Geometry: final body of the model. Coordinates: model frame, mm. A direction names the side the tool comes from. Round coordinates to 2 decimals unless told otherwise and drop trailing zeros. Write each loop counter-clockwise with the first axis right and the second up, starting at its lowest first coordinate (ties: lowest second). Pieces come first, ordered by that corner, then holes. Notation, with made-up numbers: M -28.5,22.25 L 8.5,22.25 A27 cw 8.5,61.25 Z; hole C 31.5,30.5 d2. An arc over 180 degrees is marked long. Answer as CSV lines item,"result". Start each with the question number.
Q1. Section query C-C on x = 1090.5. Output: boundary loops of the cut face in (y, z).
Q2. Reachability of faces 4 (the flat face through (1375, 624, -386)), 5 (the flat face through (419, -337, 0)), 6 (the flat face through (228, -460, -177)) from +Z, -Z, +X, -X, +Y, -Y: full face, straight path, thin tool, end or side. Return the list, or none.
Q3. Ray query, probe 1 along Y at (x, z) = (951.5, 916); probe 2 along X at (y, z) = (24, -425); probe 3 along Y at (x, z) = (288.5, -233). Return the intervals inside material, ascending.
Q4. First-contact query: pin 1 (1 mm diameter, centred on x = 1203, z = 115.5, fed in from +Y); pin 2 (12 mm diameter, centred on x = 274, y = -205.5, fed in from +Z); pin 3 (12 mm diameter, centred on x = 1136.5, y = 178.5, fed in from +Z). Flat tips, straight axial feed; report the tip coordinate or a pass-through.
Q5. Mould query, pull axis Y, two halves, no side actions, for faces 1 (the flat face through (248, -350, -350)), 2 (the flat face through (865, 40, -76)), 3 (the flat face through (1324, -710, -424)). Classes: pulls with the +Y half, pulls with the -Y half, needs draft (parallel to the pull), parting line crosses it, or undercut.
Q6. Section query B-B on x = 1325. Give the number of separate pieces and of enclosed holes in the cut face, and give its area (3 significant figures).
Q7. Section query A-A on z = 275. Output: boundary loops of the cut face in (x, y), and give its area (3 significant figures).
Q8. Section query D-D on z = -222. Output: boundary loops of the cut face in (x, y), and give its area (3 significant figures).
```python
from build123d import *

# Parameters (mm, degrees)
BOSS_EXTRUDE1_DEPTH = 40
SKETCH3_W           = 450
SKETCH3_H           = 500
SKETCH3_W_2         = 500
SKETCH3_H_2         = 450
BOSS_EXTRUDE2_DEPTH = 710
SKETCH5_W           = 410
SKETCH5_H           = 710
CUT_EXTRUDE1_DEPTH  = 150
SKETCH7_R           = 30
CUT_EXTRUDE2_DEPTH  = 150
SKETCH8_W           = 370
SKETCH8_H           = 670
CUT_EXTRUDE3_DEPTH  = 310
SKETCH9_W           = 370
SKETCH9_H           = 670
CUT_EXTRUDE4_DEPTH  = 460
SKETCH10_W          = 150
SKETCH10_H          = 150
BOSS_EXTRUDE3_DEPTH = 710
SKETCH11_W          = 310
SKETCH11_H          = 20
BOSS_EXTRUDE4_DEPTH = 410
SKETCH12_W          = 370
SKETCH12_H          = 670
CUT_EXTRUDE5_DEPTH  = 40
BOSS_EXTRUDE5_DEPTH = 370
SKETCH14_W          = 370
SKETCH14_H          = 670
CUT_EXTRUDE10_DEPTH = 40
BOSS_EXTRUDE6_DEPTH = 650
SKETCH17_W          = 175
SKETCH17_H          = 20
BOSS_EXTRUDE7_DEPTH = 1350


with BuildPart() as part:
    # Sketch2 → Boss-Extrude1 (new body)
    with BuildSketch(Plane(origin=(0, 0, 0), x_dir=(1, 0, 0), z_dir=(0, 1, 0))):
        Polygon((0, 500), (1400, 500), (900, 0), (0, 0), align=None)
        Polygon((900, 0), (1400, 500), (1400, 0), (1400, -1000), (900, -1000), align=None)
    extrude(amount=BOSS_EXTRUDE1_DEPTH)

    # Sketch3 → Boss-Extrude2 (add)
    with BuildSketch(Plane.XZ):
        with Locations((225, -250)):
            Rectangle(SKETCH3_W, SKETCH3_H)
        with Locations((1150, 775)):
            Rectangle(SKETCH3_W_2, SKETCH3_H_2)
    extrude(amount=BOSS_EXTRUDE2_DEPTH)

    # Sketch5 → Cut-Extrude1 (cut)
    with BuildSketch(Plane(origin=(0, 0, -500), x_dir=(-1, 0, 0), z_dir=(0, 0, -1))):
        with Locations((-245, -355)):
            Rectangle(SKETCH5_W, SKETCH5_H)
    extrude(amount=-CUT_EXTRUDE1_DEPTH, mode=Mode.SUBTRACT)

    # Sketch7 → Cut-Extrude2 (cut)
    with BuildSketch(Plane.XZ):
        with Locations(Location((115, -425, 0), (0, 0, 270))):
            Circle(SKETCH7_R)
        with Locations(Location((675, -425, 0), (0, 0, 270))):
            Circle(SKETCH7_R)
        with Locations(Location((1325, 275, 0), (0, 0, 270))):
            Circle(SKETCH7_R)
    extrude(amount=-CUT_EXTRUDE2_DEPTH, mode=Mode.SUBTRACT)

    # Sketch8 → Cut-Extrude3 (cut)
    with BuildSketch(Plane.XY):
        with Locations((225, -335)):
            Rectangle(SKETCH8_W, SKETCH8_H)
    extrude(amount=-CUT_EXTRUDE3_DEPTH, mode=Mode.SUBTRACT)

    # Sketch9 → Cut-Extrude4 (cut)
    with BuildSketch(Plane.ZY.offset(-900)):
        with Locations((775, -335)):
            Rectangle(SKETCH9_W, SKETCH9_H)
    extrude(amount=-CUT_EXTRUDE4_DEPTH, mode=Mode.SUBTRACT)

    # Sketch10 → Boss-Extrude3 (add)
    with BuildSketch(Plane.XZ):
        with Locations((1325, 75)):
            Rectangle(SKETCH10_W, SKETCH10_H)
        with Locations((1325, -425)):
            Rectangle(SKETCH10_W, SKETCH10_H)
    extrude(amount=BOSS_EXTRUDE3_DEPTH)

    # Sketch11 → Boss-Extrude4 (add)
    with BuildSketch(Plane.ZY.offset(-410)):
        with Locations((-155, -220)):
            Rectangle(SKETCH11_W, SKETCH11_H)
        with Locations((-155, -450)):
            Rectangle(SKETCH11_W, SKETCH11_H)
    extrude(amount=BOSS_EXTRUDE4_DEPTH)

    # Sketch12 → Cut-Extrude5 (cut)
    with BuildSketch(Plane.XY):
        with Locations((225, -335)):
            Rectangle(SKETCH12_W, SKETCH12_H)
    extrude(amount=-CUT_EXTRUDE5_DEPTH, mode=Mode.SUBTRACT)

    # Sketch13 → Boss-Extrude5 (add)
    with BuildSketch(Plane.XY.offset(590)):
        Polygon((1360, -320), (900, -320), (900, -335), (900, -350), (1360, -350), align=None)
    extrude(amount=BOSS_EXTRUDE5_DEPTH)

    # Sketch14 → Cut-Extrude10 (cut)
    with BuildSketch(Plane.ZY.offset(-900)):
        with Locations((775, -335)):
            Rectangle(SKETCH14_W, SKETCH14_H)
    extrude(amount=-CUT_EXTRUDE10_DEPTH, mode=Mode.SUBTRACT)

    # Sketch16 → Boss-Extrude6 (add)
    with BuildSketch(Plane(origin=(0, 40, 0), x_dir=(1, 0, 0), z_dir=(0, 1, 0))):
        Polygon((0, 500), (1400, 500), (1400, 300), (1375, 300), (1375, 475), (25, 475), (25, 300), (0, 300), align=None)
    extrude(amount=BOSS_EXTRUDE6_DEPTH)

    # Sketch17 → Boss-Extrude7 (add)
    with BuildSketch(Plane(origin=(25, 0, 0), x_dir=(0, 0, -1), z_dir=(1, 0, 0))):
        with Locations((387.5, 550)):
            Rectangle(SKETCH17_W, SKETCH17_H)
    extrude(amount=BOSS_EXTRUDE7_DEPTH)


solid = part.part
```
Entries:
1,outline,"M -710,550 L 0,550 L 0,-500 L 690,-500 L 690,-475 L 560,-475 L 560,-300 L 540,-300 L 540,-475 L 40,-475 L 40,1000 L -710,1000 Z; hole M -670,590 L -350,590 L -350,960 L -670,960 Z; hole M -320,590 L 0,590 L 0,960 L -320,960 Z"
2,face 4,"+Z, +Y"
2,face 5,"+Z, -X, +Y, -Y"
2,face 6,"+Z"
3,probe 1,"y = -710 to -670, -350 to -320, 0 to 40"
3,probe 2,"x = 0 to 85, 145 to 645, 705 to 1400"
3,probe 3,"y = -710 to -670, -460 to -440, -230 to -210, 0 to 40"
4,pin 1,"stops at y = 40"
4,pin 2,"stops at z = -40"
4,pin 3,"stops at z = -475"
5,face 1,"needs draft"
5,face 2,"undercut"
5,face 3,"pulls with the -Y half"
6,separate pieces,"2"
6,enclosed holes,"2"
6,area,"373,000 mm^2"
7,outline,"M 900,0 L 1295,0 L 1295,40 L 900,40 Z; M 1355,0 L 1400,0 L 1400,40 L 1355,40 Z"
7,area,"17,600 mm^2"
8,outline,"M 0,-710 L 450,-710 L 450,0 L 1400,0 L 1400,40 L 0,40 Z; hole M 40,-670 L 410,-670 L 410,-460 L 40,-460 Z; hole M 40,-440 L 410,-440 L 410,-230 L 40,-230 Z; hole M 40,-210 L 410,-210 L 410,0 L 40,0 Z"
8,area,"142,000 mm^2"
